from build123d import *

# Parameters (mm, degrees)
EXTRUDE1_DEPTH = 13
SKETCH3_R      = 2.15
EXTRUDE2_DEPTH = 30
EXTRUDE3_START = -4
EXTRUDE3_DEPTH = 30


with BuildPart() as part:
    # Sketch2 → Extrude1 (new body)
    with BuildSketch(Plane(origin=(0, 0, 0), x_dir=(0, 0, -1), z_dir=(1, 0, 0))):
        with BuildLine():
            Line((0, 0), (18, 0))
            ThreePointArc((18, 0), (12.727922061, 12.727922061), (0, 18))
            Line((0, 18), (0, 0))
        make_face()
    extrude(amount=EXTRUDE1_DEPTH)

    # Sketch3 → Extrude2 (cut)
    with BuildSketch(Plane.XY):
        with Locations((6.5, 11.5)):
            Circle(SKETCH3_R)
    extrude2 = extrude(amount=-EXTRUDE2_DEPTH, mode=Mode.SUBTRACT)

    # Sketch5 → Extrude3 (cut)
    with BuildSketch(Plane.XY.offset(EXTRUDE3_START)):
        Polygon((6.5, 15.656921938), (2.9, 13.578460969), (2.9, 9.421539031), (6.5, 7.343078062), (10.1, 9.421539031), (10.1, 13.578460969), align=None)
    extrude3 = extrude(amount=-EXTRUDE3_DEPTH, mode=Mode.SUBTRACT)

    # Mirror1: Extrude2, Extrude3 across plane
    add(extrude2.mirror(Plane(origin=(0, 0, 0), x_dir=(0, -0.707106781, 0.707106781), z_dir=(0, 0.707106781, 0.707106781))), mode=Mode.SUBTRACT)
    add(extrude3.mirror(Plane(origin=(0, 0, 0), x_dir=(0, -0.707106781, 0.707106781), z_dir=(0, 0.707106781, 0.707106781))), mode=Mode.SUBTRACT)


solid = part.part
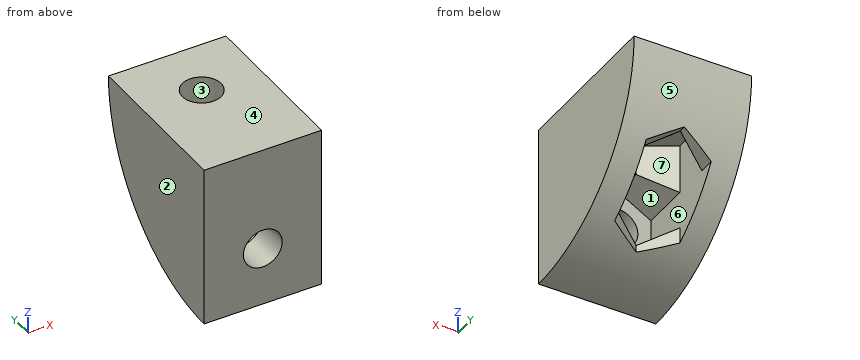
Check sheet for the modelled part. Datum: model origin and axes. Units: mm. Face numbers are marked on the shaded views. A direction names the side the tool comes from. Coordinates: 2 decimals unless noted, no trailing zeros. Write each loop counter-clockwise with the first axis right and the second up, starting at its lowest first coordinate (ties: lowest second). Pieces come first, ordered by that corner, then holes. Notation, with made-up numbers: M 24,85.25 L 74,85.25 A9 cw 74,102.25 Z; hole C 59.25,84.25 d7. An arc over 180 degrees is marked long. Answer as CSV lines item,"result".
Q1. Cross-section at A-A (y = 11.5). Record the boundary of the cut face in (x, z).
Check result:
outline,"M 0,-13.85 L 2.9,-13.85 L 2.9,-4 L 4.35,-4 L 4.35,0 L 0,0 Z; M 8.65,-4 L 10.1,-4 L 10.1,-13.85 L 13,-13.85 L 13,0 L 8.65,0 Z"
Q2. Cross-section at B-B (z = -13.25). Record the boundary of the cut face in (x, y).
Check result:
outline,"M 0,0 L 5.25,0 L 5.25,4 L 2.9,4 L 2.9,12.18 L 0,12.18 Z; M 7.75,0 L 13,0 L 13,12.18 L 10.1,12.18 L 10.1,4 L 7.75,4 Z"
Q3. Go/stop test with flat-tipped pins: pin 1 (5 mm diameter, centred on x = 6.5, z = -11.5, fed in from -Y); pin 2 (6 mm diameter, centred on x = 7.5, y = 11.5, fed in from -Z); pin 3 (1 mm diameter, centred on x = 3.5, y = 2.5, fed in from -Z); pin 4 (3.5 mm diameter, centred on x = 8, z = -12, fed in from +Y). Record where each tip stops, or that it passes through.
Check result:
pin 1,"y = 0"
pin 2,"z = -14.96"
pin 3,"z = -17.89"
pin 4,"y = 4"
Q4. Cross-section at D-D (y = 2.75). Record the boundary of the cut face in (x, z), then the cut area to 3 significant figures.
Check result:
outline,"M 0,-17.79 L 13,-17.79 L 13,0 L 0,0 Z; hole C 6.5,-11.5 d4.3"
area,"217 mm^2"
Q5. Set-up check for the marked faces 5, 6 and 7: record each of +Z, -Z, +X, -X, +Y, -Y from which the full face is reachable in a straight line by a thin tool's end or side.
Check result:
face 5,"-Z, +X, -X, +Y"
face 6,"none"
face 7,"-Z"
Q6. Material ranges on probe 1 along X at (y, z) = (11.25, -14); probe 2 along X at (y, z) = (2.4, -11.5); probe 3 along Y at (x, z) = (8.25, -8.75), recorded low to high. Write a range as from..to.
Check result:
probe 1,"0..2.9, 10.1..13"
probe 2,"0..4.35, 8.65..13"
probe 3,"0..4"
Q7. Mould release check, pull along X, two halves, no side actions. Record for the marked faces 1, 2, 3 and 4: released by +X, released by -X, zero draft, split by the parting line, or undercut.
Check result:
face 1,"undercut"
face 2,"released by -X"
face 3,"undercut"
face 4,"zero draft"
Q8. Cross-section at C-C (x = 6.25). Record the boundary of the cut face in (y, z), then the cut area to 3 significant figures.
Check result:
outline,"M 0,-18 A18 ccw 7.49,-16.37 L 7.49,-15.51 L 4,-15.51 L 4,-13.64 L 0,-13.64 Z; M 0,-9.36 L 4,-9.36 L 4,-7.49 L 7.49,-7.49 L 7.49,-4 L 9.36,-4 L 9.36,0 L 0,0 Z; M 13.64,-4 L 15.51,-4 L 15.51,-7.49 L 16.37,-7.49 A18 ccw 18,0 L 13.64,0 Z"
area,"115 mm^2"
